```python
from build123d import *

# Parameters (mm, degrees)
F1_DEPTH = 1500


with BuildPart() as f1:
    # F0 (on Front) → F1 (new body)
    with BuildSketch(Plane.XZ):
        with BuildLine():
            Line((0, 70.887234), (0, 90))
            ThreePointArc((0, 90), (-63.63961, 63.63961), (-90, 0))
            Line((-90, 0), (-70.887234, 0))
            Line((-70.887234, 0), (-70.887234, 10))
            Line((-70.887234, 10), (-22.813418, 19.481991))
            ThreePointArc((-22.813418, 19.481991), (-21.213203, 21.213203), (-19.481991, 22.813418))
            Line((-19.481991, 22.813418), (-10, 70.887234))
            Line((-10, 70.887234), (0, 70.887234))
        make_face()
    extrude(amount=-F1_DEPTH)


solid = f1.part
```
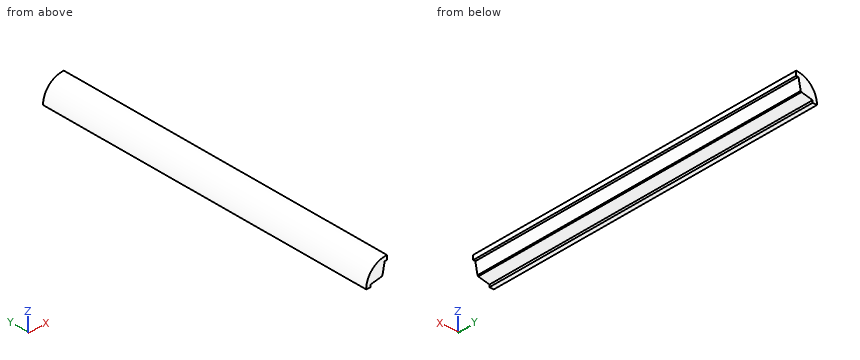
Input: part model. Units: mm. Frame: model coordinates. Coordinates: 2 decimals unless noted, no trailing zeros. Loops run counter-clockwise (first coordinate to the right, second up) from the corner with the lowest first, then second, coordinate; pieces in that order, holes last.
Q1. Section B-B, the plane z = 50. Return the cut outline in (x, y).
Results are:
outline: (-74.83, 0) - (-14.12, 0) - (-14.12, 1500) - (-74.83, 1500) - close
Q2. Section A-A, the plane y = 278.5. Return the cut outline in (x, z).
Results are:
outline: (-90, 0) - (-70.89, 0) - (-70.89, 10) - (-22.81, 19.48) arc R30 cw to (-19.48, 22.81) - (-10, 70.89) - (0, 70.89) - (0, 90) arc R90 ccw to start
Q3. Section C-C, the plane x = -44. Return the cut outline in (y, z).
Results are:
outline: (0, 15.3) - (1500, 15.3) - (1500, 78.51) - (0, 78.51) - close
Q4. Contact query for flat-ended pins moving along their axis: pin 1 (10 mm diameter, centred on x = -53, y = 406.5, fed in from -Z); pin 2 (11 mm diameter, centred on x = -4, y = 423, fed in from -Z); pin 3 (10 mm diameter, centred on x = -52.5, y = 1235, fed in from +Z); pin 4 (5 mm diameter, centred on x = -41.5, z = 41, fed in from -Y). Output: stop coordinate, or through.
Results are:
pin 1: stops at z = 12.54
pin 2: stops at z = 70.89
pin 3: stops at z = 76.44
pin 4: stops at y = 0
Q5. Line query: line 1 along X through (y, z) = (178, 4); line 2 along Z through (x, y) = (-53, 1091.5); line 3 along X through (y, z) = (359, 62). Output: solid intervals per line, ascending.
Results are:
line 1: x = -89.91 to -70.89
line 2: z = 13.53 to 72.74
line 3: x = -65.24 to -11.75
